from build123d import *

# Parameters (mm, degrees)
CROQUIS1_R                 = 4
SALIENTE_EXTRUIR2_DEPTH    = 15
CROQUIS2_R                 = 7.5
CROQUIS2_R_2               = 4
SALIENTE_EXTRUIR3_DEPTH    = 10
CROQUIS3_R                 = 4.006471319
CROQUIS3_R_2               = 4.004031771
SALIENTE_EXTRUIR4_DEPTH    = 2
CROQUIS4_R                 = 1.5
CORTAR_EXTRUIR1_DEPTH      = 6
CROQUIS5_W                 = 8
CROQUIS5_H                 = 4
CORTAR_EXTRUIR2_DEPTH      = 15
CORTAR_EXTRUIR2_DEPTH_BACK = 2.5


with BuildPart() as part:
    # Croquis1 → Saliente-Extruir2 (new body)
    with BuildSketch(Plane.XY):
        with BuildLine():
            Line((28.5, 85.161764706), (28.5, 47.838235294))
            Line((28.5, 47.838235294), (11.5, 47.838235294))
            Line((11.5, 47.838235294), (11.5, 44.838235294))
            Line((11.5, 44.838235294), (9.5, 44.838235294))
            Line((9.5, 44.838235294), (9.5, 47.838235294))
            Line((9.5, 47.838235294), (1.067079587, 47.838235294))
            Line((1.067079587, 47.838235294), (-8.503797206, 25.875519531))
            ThreePointArc((-8.503797206, 25.875519531), (-18.751450015, 17.08519644), (-5.5, 14.5))
            Line((-5.5, 14.5), (25.080237482, 14.5))
            Line((25.080237482, 14.5), (33.5, 12.617754504))
            Line((33.5, 12.617754504), (33.5, 4.5))
            Line((33.5, 4.5), (38.5, 4.5))
            Line((38.5, 4.5), (38.5, 11.5))
            Line((38.5, 11.5), (38.5, 121.5))
            Line((38.5, 121.5), (38.5, 128.5))
            Line((38.5, 128.5), (33.5, 128.5))
            Line((33.5, 128.5), (33.5, 120.382245496))
            Line((33.5, 120.382245496), (25.080237482, 118.5))
            Line((25.080237482, 118.5), (-5.5, 118.5))
            ThreePointArc((-5.5, 118.5), (-18.751450015, 115.91480356), (-8.503797206, 107.124480469))
            Line((-8.503797206, 107.124480469), (1.067079587, 85.161764706))
            Line((1.067079587, 85.161764706), (9.5, 85.161764706))
            Line((9.5, 85.161764706), (9.5, 88.161764706))
            Line((9.5, 88.161764706), (11.5, 88.161764706))
            Line((11.5, 88.161764706), (11.5, 85.161764706))
            Line((11.5, 85.161764706), (28.5, 85.161764706))
        make_face()
        with Locations((-11.5, 114)):
            Circle(CROQUIS1_R, mode=Mode.SUBTRACT)
        with Locations((-11.5, 19)):
            Circle(CROQUIS1_R, mode=Mode.SUBTRACT)
        Polygon((28.5, 22.676470588), (28.5, 40.838235294), (12.25, 40.838235294), align=None, mode=Mode.SUBTRACT)
        Polygon((28.5, 110.323529412), (28.5, 92.161764706), (12.25, 92.161764706), align=None, mode=Mode.SUBTRACT)
        Polygon((25.080237482, 114), (5.540763798, 92.161764706), (5.540763798, 114), align=None, mode=Mode.SUBTRACT)
        Polygon((5.540763798, 40.838235294), (25.080237482, 19), (5.540763798, 19), align=None, mode=Mode.SUBTRACT)
    extrude(amount=SALIENTE_EXTRUIR2_DEPTH)

    # Croquis2 → Saliente-Extruir3 (add)
    with BuildSketch(Plane.XY.offset(15)):
        with Locations((-11.5, 114)):
            Circle(CROQUIS2_R)
        with Locations((-11.5, 114)):
            Circle(CROQUIS2_R_2, mode=Mode.SUBTRACT)
        with Locations((-11.5, 19)):
            Circle(CROQUIS2_R)
        with Locations((-11.5, 19)):
            Circle(CROQUIS2_R_2, mode=Mode.SUBTRACT)
    extrude(amount=SALIENTE_EXTRUIR3_DEPTH)

    # Croquis3 → Saliente-Extruir4 (add)
    with BuildSketch(Plane(origin=(0, 0, 0), x_dir=(-1, 0, 0), z_dir=(0, 0, -1))):
        with Locations((11.5, 114)):
            Circle(CROQUIS3_R)
        with Locations((11.5, 19)):
            Circle(CROQUIS3_R_2)
    extrude(amount=-SALIENTE_EXTRUIR4_DEPTH)

    # Croquis4 → Cortar-Extruir1 (cut, through all)
    with BuildSketch(Plane.ZY.offset(-33.5)):
        with Locations((5, 125)):
            Circle(CROQUIS4_R)
        with Locations((5, 8)):
            Circle(CROQUIS4_R)
    extrude(amount=-CORTAR_EXTRUIR1_DEPTH, mode=Mode.SUBTRACT)

    # Croquis5 → Cortar-Extruir2 (cut, two sides)
    with BuildSketch(Plane.ZY.offset(-11.5)) as cortar_extruir2_sk:
        with Locations((7.5, 87.161764706)):
            Rectangle(CROQUIS5_W, CROQUIS5_H)
        with Locations((7.5, 45.838235294)):
            Rectangle(CROQUIS5_W, CROQUIS5_H)
    extrude(amount=CORTAR_EXTRUIR2_DEPTH, mode=Mode.SUBTRACT)
    extrude(cortar_extruir2_sk.sketch, amount=-CORTAR_EXTRUIR2_DEPTH_BACK, mode=Mode.SUBTRACT)


solid = part.part
Geometry: final body of the model. Coordinates: model frame, mm. A direction names the side the tool comes from. Give positions to 0.01 mm unless a question says otherwise; leave off trailing zeros. Write each loop counter-clockwise with the first axis right and the second up, starting at its lowest first coordinate (ties: lowest second). Pieces come first, ordered by that corner, then holes. Notation, with made-up numbers: (-36.75, 55.25) -> (-25.75, 55.25) arc R17 cw to (-25.75, 69.25) -> close; hole circle Ø7 at (-31.5, -17). An arc over 180 degrees is marked (long way). Answer as a JSON object with one key per item and string values.
1. Ray query, probe 1 along Y at (x, z) = (-11.5, 15.5); probe 2 along Y at (x, z) = (35, 5); probe 3 along Z at (x, y) = (35.25, 125). Return the intervals inside material, ascending. Write a range as from..to.
Ans:
{"probe 1": "y = 11.5..15, 23..26.5, 106.5..110, 118..121.5", "probe 2": "y = 4.5..6.5, 9.5..123.5, 126.5..128.5", "probe 3": "z = 0..3.5, 6.5..15"}
2. Access query for faces 4 (the flat face through (7, 46, 11.5)), 5 (the flat face through (5, 47.838, 13)), 6 (the flat face through (28.5, 32, 7)). Directions: +Z, -Z, +X, -X, +Y, -Y. A direction counts if a zero-diameter tool reaches every point of the face in a straight line with its end or side. Return the directions, or none.
Ans:
{"face 4": "-X", "face 5": "+Z, -Z, -X", "face 6": "+Z, -Z"}
3. Mould query, pull axis Z, two halves, no side actions, for faces 1 (the flat face through (14, 46, 7)), 2 (the flat face through (-3.785, 96.297, 7.395)), 3 (the flat face through (-11, 114, 2)). Classes: pulls with the +Z half, pulls with the -Z half, needs draft (parallel to the pull), parting line crosses it, or undercut.
Ans:
{"face 1": "undercut", "face 2": "needs draft", "face 3": "pulls with the +Z half"}
4. Cut plane D-D on x = 8. Output: boundary loops of the cut face in (y, z).
Ans:
{"outline": "(14.5, 0) -> (19, 0) -> (19, 15) -> (14.5, 15) -> close; (38.09, 0) -> (47.84, 0) -> (47.84, 3.5) -> (43.84, 3.5) -> (43.84, 11.5) -> (47.84, 11.5) -> (47.84, 15) -> (38.09, 15) -> close; (85.16, 0) -> (94.91, 0) -> (94.91, 15) -> (85.16, 15) -> (85.16, 11.5) -> (89.16, 11.5) -> (89.16, 3.5) -> (85.16, 3.5) -> close; (114, 0) -> (118.5, 0) -> (118.5, 15) -> (114, 15) -> close"}
5. Cut plane B-B on z = 9.75. Count the separate pieces of the cut face and the enclosed holes in it, and give its area (3 significant figures).
Ans:
{"separate pieces": "1", "enclosed holes": "6", "area": "2,750 mm^2"}
6. Cut plane A-A on y = 8. Output: boundary loops of the cut face in (x, z).
Ans:
{"outline": "(33.5, 0) -> (38.5, 0) -> (38.5, 3.5) -> (33.5, 3.5) -> close; (33.5, 6.5) -> (38.5, 6.5) -> (38.5, 15) -> (33.5, 15) -> close"}
7. Cut plane C-C on y = 97.5. Output: boundary loops of the cut face in (x, z), and give its area (3 significant figures).
Ans:
{"outline": "(-4.31, 0) -> (5.54, 0) -> (5.54, 15) -> (-4.31, 15) -> close; (10.32, 0) -> (17.03, 0) -> (17.03, 15) -> (10.32, 15) -> close; (28.5, 0) -> (38.5, 0) -> (38.5, 15) -> (28.5, 15) -> close", "area": "398 mm^2"}
8. Contact query for flat-ended pins moving along their axis: pin 1 (4.5 mm diameter, centred on x = 24, z = 10.5, fed in from -Y); pin 2 (12 mm diameter, centred on x = 6, y = 115, fed in from +Z); pin 3 (1.5 mm diameter, centred on x = 22, z = 4, fed in from -Y). Output: stop coordinate, or through.
Ans:
{"pin 1": "stops at y = 14.24", "pin 2": "stops at z = 15", "pin 3": "stops at y = 14.5"}
